from build123d import *

# Parameters (mm, degrees)
SKETCH_W        = 125
SKETCH_H        = 88
PAD_DEPTH       = 32
SKETCH001_W     = 120
SKETCH001_H     = 83
POCKET_DEPTH    = 32
SKETCH002_R     = 6
PAD001_DEPTH    = 30
SKETCH003_R     = 5.25
POCKET001_DEPTH = 2
FILLET_R        = 2.5
FILLET001_R     = 2.5
FILLET002_R     = 2.5
FILLET003_R     = 2.5
FILLET004_R     = 5
FILLET005_R     = 5
FILLET006_R     = 5
FILLET007_R     = 5
SKETCH004_R     = 10.125
POCKET002_DEPTH = 1


with BuildPart() as part:
    # Sketch → Pad (new body)
    with BuildSketch(Plane.XY):
        with Locations((62.5, 44)):
            Rectangle(SKETCH_W, SKETCH_H)
    extrude(amount=PAD_DEPTH)

    # Sketch001 → Pocket (cut)
    with BuildSketch(Plane.XY.offset(34)):
        with Locations((62.5, 44)):
            Rectangle(SKETCH001_W, SKETCH001_H)
    extrude(amount=-POCKET_DEPTH, mode=Mode.SUBTRACT)

    # Sketch002 (on Face11 of Pocket) → Pad001 (join)
    with BuildSketch(Plane.XY.offset(2)):
        with Locations((6, 6)):
            Circle(SKETCH002_R)
        with Locations((6, 82)):
            Circle(SKETCH002_R)
        with Locations((119, 82)):
            Circle(SKETCH002_R)
        with Locations((119, 6)):
            Circle(SKETCH002_R)
    extrude(amount=PAD001_DEPTH)

    # Sketch003 (on Face27 of Pad001) → Pocket001 (cut)
    with BuildSketch(Plane.XY.offset(32)):
        with Locations((6, 6)):
            Circle(SKETCH003_R)
        with Locations((6, 82)):
            Circle(SKETCH003_R)
        with Locations((119, 82)):
            Circle(SKETCH003_R)
        with Locations((119, 6)):
            Circle(SKETCH003_R)
    extrude(amount=-POCKET001_DEPTH, mode=Mode.SUBTRACT)

    # Fillet
    fillet_edges = [part.edges().sort_by_distance(p)[0] for p in [
        (62.5, 2.5, 2),
    ]]
    fillet(fillet_edges, radius=FILLET_R)

    # Fillet001
    fillet001_edges = [part.edges().sort_by_distance(p)[0] for p in [
        (122.5, 44, 2),
    ]]
    fillet(fillet001_edges, radius=FILLET001_R)

    # Fillet002
    fillet002_edges = [part.edges().sort_by_distance(p)[0] for p in [
        (62.5, 85.5, 2),
    ]]
    fillet(fillet002_edges, radius=FILLET002_R)

    # Fillet003
    fillet003_edges = [part.edges().sort_by_distance(p)[0] for p in [
        (2.5, 44, 2),
    ]]
    fillet(fillet003_edges, radius=FILLET003_R)

    # Fillet004
    fillet004_edges = [part.edges().sort_by_distance(p)[0] for p in [
        (125, 88, 16),
    ]]
    fillet(fillet004_edges, radius=FILLET004_R)

    # Fillet005
    fillet005_edges = [part.edges().sort_by_distance(p)[0] for p in [
        (125, 0, 16),
    ]]
    fillet(fillet005_edges, radius=FILLET005_R)

    # Fillet006
    fillet006_edges = [part.edges().sort_by_distance(p)[0] for p in [
        (0, 0, 16),
    ]]
    fillet(fillet006_edges, radius=FILLET006_R)

    # Fillet007
    fillet007_edges = [part.edges().sort_by_distance(p)[0] for p in [
        (0, 88, 16),
    ]]
    fillet(fillet007_edges, radius=FILLET007_R)

    # Sketch004 (on Face6 of Fillet007) → Pocket002 (cut)
    with BuildSketch(Plane.XZ):
        with Locations((62.5, 16)):
            Circle(SKETCH004_R)
    extrude(amount=-POCKET002_DEPTH, mode=Mode.SUBTRACT)


solid = part.part
Here's how the part is built. I have some questions about the finished solid (model axes, mm). A direction names the side the tool comes from. Round coordinates to 2 decimals unless told otherwise and drop trailing zeros. Order: outer loops, then holes, each group sorted by start corner. A loop starts at its lowest first (then second) coordinate and runs counter-clockwise, first axis right, second up. Notation, with made-up numbers: (-13, -6.75) -> (28, -6.75) arc R34 ccw to (28, 28.25) -> close; hole circle Ø3 at (-6, 25.5). An arc over 180 degrees is marked (long way). Use CSV: the item, a comma, the result in double quotes.
1. Which directions (+Z, -Z, +X, -X, +Y, -Y) give clear straight access to the entire face, cutting with the end or side of a thin tool? Please do faces 4 (the face through (72.157, 0.493, 19.041)), 5 (the face through (124, 2, 16)), 6 (the face through (63, 3, 3)).
Recorded:
face 4,"-Y"
face 5,"+Z, -Z, +X, -Y"
face 6,"+Z"
2. I want a section at D-D on z = 9. List the corners of the cut face in (x, y) for me, and give its area (3 significant figures).
Recorded:
outline,"(0, 5) arc R5 ccw to (5, 0) -> (55.18, 0) -> (55.18, 1) -> (69.82, 1) -> (69.82, 0) -> (120, 0) arc R5 ccw to (125, 5) -> (125, 83) arc R5 ccw to (120, 88) -> (5, 88) arc R5 ccw to (0, 83) -> close; hole (2.5, 10.87) arc R6 cw to (10.87, 2.5) -> (114.13, 2.5) arc R6 cw to (122.5, 10.87) -> (122.5, 77.13) arc R6 cw to (114.13, 85.5) -> (10.87, 85.5) arc R6 cw to (2.5, 77.13) -> close"
area,"1,320 mm2"
3. I want a section at C-C on y = 45.5. List the corners of the cut face in (x, z) for me, and give its area (3 significant figures).
Recorded:
outline,"(0, 0) -> (125, 0) -> (125, 32) -> (122.5, 32) -> (122.5, 4.5) arc R2.5 cw to (120, 2) -> (5, 2) arc R2.5 cw to (2.5, 4.5) -> (2.5, 32) -> (0, 32) -> close"
area,"403 mm2"
4. I'm going to push flat-ended pins straight in: P1, Ø3, axis at x = 117, y = 5, coming from the +Z side; P2, Ø18, axis at x = 62.5, z = 16, coming from the -Y side; P3, Ø2, axis at x = 67, y = 40.5, coming from the +Z side. Where does each tip first touch, or does it pass through?
Recorded:
P1,"stops at z = 30"
P2,"stops at y = 1"
P3,"stops at z = 2"
5. I need wall thicknesses on line 1 along Y through (x, z) = (119, 30.9); line 2 along Y through (x, z) = (38, 8); line 3 along Z through (x, y) = (62.5, 0.25) (3 decimals). Which ranges of each line are inside material? Lowest first, please.
Recorded:
line 1,"y = 0 to 0.75, 11.25 to 12, 76 to 76.75, 87.25 to 88"
line 2,"y = 0 to 2.5, 85.5 to 88"
line 3,"z = 0 to 5.875, 26.125 to 32"
6. I want a section at A-A on z = 16. List the corners of the cut face in (x, y) for me (3 decimals).
Recorded:
outline,"(0, 5) arc R5 ccw to (5, 0) -> (52.375, 0) -> (52.375, 1) -> (72.625, 1) -> (72.625, 0) -> (120, 0) arc R5 ccw to (125, 5) -> (125, 83) arc R5 ccw to (120, 88) -> (5, 88) arc R5 ccw to (0, 83) -> close; hole (2.5, 10.873) arc R6 cw to (10.873, 2.5) -> (114.127, 2.5) arc R6 cw to (122.5, 10.873) -> (122.5, 77.127) arc R6 cw to (114.127, 85.5) -> (10.873, 85.5) arc R6 cw to (2.5, 77.127) -> close"
7. Thinking about a two-plate mould opening in X: for faces 1 (the face through (44, 2, 32)), 2 (the face through (125, 43, 16)), 3 (the face through (114.675, 77.842, 16.79)), which applies, pulls with the +X half, pulls with the -X half, needs draft (parallel to the pull), parting line crosses it, or undercut?
Recorded:
face 1,"needs draft"
face 2,"pulls with the +X half"
face 3,"undercut"
8. I want a section at B-B on x = 18. List the corners of the cut face in (y, z) for me, and give its area (3 significant figures).
Recorded:
outline,"(0, 0) -> (88, 0) -> (88, 32) -> (85.5, 32) -> (85.5, 4.5) arc R2.5 cw to (83, 2) -> (5, 2) arc R2.5 cw to (2.5, 4.5) -> (2.5, 32) -> (0, 32) -> close"
area,"329 mm2"
